Autodesk Inventor part; units mm, degrees
ref_plane "YZ Plane" through (0, 0, 0) normal (1, 0, 0) x (0, 1, 0)
ref_plane "XZ Plane" through (0, 0, 0) normal (0, 1, 0) x (-1, 0, 0)
ref_plane "XY Plane" through (0, 0, 0) normal (0, 0, 1) x (1, 0, 0)
sketch "Sketch1" plane through (0, 0, 0) normal (0, 1, 0) x (-1, 0, 0)
  line L0 (15, 35) -> (-15, 35)
  line L1 (-15, 35) -> (-15, -35)
  line L2 (-15, -35) -> (15, -35)
  line L3 (15, -35) -> (15, 35)
  line L4 (15, 35) -> (-15, -35) construction
  line L5 (-15, 35) -> (15, -35) construction
  point P0 (0, 0)
  dimension "d0" = 30
  dimension "d1" = 70
extrude "gabaryty" add sketch "Sketch1" along normal blind 10
sketch "Sketch2" plane through (0, 10, 0) normal (0, 1, 0) x (1, 0, 0)
  line L0 (5.2, -26) -> (-5.2, -26)
  line L1 (-5.2, -26) -> (-5.2, 26)
  line L2 (-5.2, 26) -> (5.2, 26)
  line L3 (5.2, 26) -> (5.2, -26)
  line L4 (5.2, -26) -> (-5.2, 26) construction
  line L5 (-5.2, -26) -> (5.2, 26) construction
  point P0 (0, 0)
  dimension "d4" = 10.4
  dimension "d5" = 52
extrude "przestrzen srodek" cut sketch "Sketch2" against normal through all
sketch "Sketch3" plane through (0, 10, 0) normal (0, 1, 0) x (1, 0, 0)
  line L0 (5, 5) -> (-5, 5)
  line L1 (-5, 5) -> (-5, -5)
  line L2 (-5, -5) -> (5, -5)
  line L3 (5, -5) -> (5, 5)
  line L4 (5, 5) -> (-5, -5) construction
  line L5 (-5, 5) -> (5, -5) construction
  point P0 (0, 0)
  dimension "d8" = 10
  dimension "d9" = 10
extrude "bloczek srodek" add sketch "Sketch3" against normal blind 10
sketch "Sketch4" plane through (0, 10, 0) normal (0, 1, 0) x (1, 0, 0)
  line L0 (-5, 5) -> (-5, -5) construction
  line L1 (-5, -5) -> (5, -5) construction
  line L2 (5, -5) -> (5, 5) construction
  line L3 (5, 5) -> (-5, 5) construction
  line L4 (-5.2, -26) -> (-5.2, 26) construction
  line L5 (-5.2, 26) -> (5.2, 26) construction
  line L6 (5.2, 26) -> (5.2, -26) construction
  line L7 (5.2, -26) -> (-5.2, -26) construction
  line L8 (15, -35) -> (15, 35) construction
  line L9 (15, 35) -> (-15, 35) construction
  line L10 (-15, 35) -> (-15, -35) construction
  line L11 (-15, -35) -> (15, -35) construction
  line L12 (-5.2, -26) -> (5.2, -26)
  line L13 (-3, -5) -> (-2.6, -5)
  line L14 (-2.6, -5) -> (-2.6, -26)
  line L15 (-2.6, -26) -> (-3, -26)
  line L16 (-3, -26) -> (-3, -5)
  line L17 (3, -5) -> (2.6, -5)
  line L18 (2.6, -5) -> (2.6, -26)
  line L19 (2.6, -26) -> (3, -26)
  line L20 (3, -26) -> (3, -5)
  line L21 (3, 5) -> (2.6, 5)
  line L22 (2.6, 5) -> (2.6, 26)
  line L23 (2.6, 26) -> (3, 26)
  line L24 (3, 26) -> (3, 5)
  line L25 (-5, 5) -> (5, 5)
  line L26 (-3, 5) -> (-2.6, 5)
  line L27 (-2.6, 5) -> (-2.6, 26)
  line L28 (-2.6, 26) -> (-3, 26)
  line L29 (-3, 26) -> (-3, 5)
  point P0 (0, 0)
  point P1 (-2.6, 5)
  dimension "d12" = 0.4
  dimension "d13" = 2
  dimension "d14" = 0.4
  dimension "d15" = 2
  dimension "d16" = 0.4
  dimension "d17" = 2
  dimension "d18" = 0.4
  dimension "d19" = 2
extrude "Belki" add sketch "Sketch4" against normal blind 10
sketch "Sketch5" plane through (0, 10, 0) normal (0, 1, 0) x (1, 0, 0)
  point P0 (0, 0)
  point P1 (0, 0)
hole "srodek" at (0, 10, 0) direction (0, -1, 0) diameter 5.5 end through all
sketch "Sketch6" plane through (-15, 0, -35) normal (-1, 0, 0) x (0, 0, 1)
  line L0 (0, 0) -> (70, 0) construction
  line L1 (70, 0) -> (70, 10) construction
  line L2 (0, 10) -> (70, 10) construction
  line L3 (0, 0) -> (0, 10) construction
  line L4 (35, 0) -> (35, 10) construction
  point P0 (45, 5)
  point P1 (25, 5)
  dimension "d29" = 10
  dimension "d30" = 10
  dimension "d31" = 5
  dimension "d32" = 5
hole "mocowanie gora" at (-15, 5, 10) at (-15, 5, -10) direction (1, 0, 0) diameter 2.459 depth 9.8
chamfer "Chamfer1" distance 0.5 angle 45 2 edges at (-15, 5, -11.2295) (-15, 5, 8.7705)
fillet "zaokraglenie lasera" radius 0.1 24 edges at (-3, 5, 5) (-2.6, 5, 5) (-3, 5, 26) (-2.6, 5, 26) (2.6, 5, 26) (2.6, 5, 5) (3, 5, 5) (3, 5, 26) (3, 5, -5) (2.6, 5, -5) (-2.6, 5, -5) (-3, 5, -5) (-3, 5, -26) (2.6, 5, -26) (-2.6, 5, -26) (3, 5, -26) (-5.2, 5, 26) (-5.2, 5, -26) (5.2, 5, -26) (5.2, 5, 26) (-5, 5, 5) (-5, 5, -5) (5, 5, -5) (5, 5, 5)
chamfer "Chamfer2" distance 0.2 angle 45 1 edges at (0, 10, -2.75)
equation "\"d14\" = d12"
equation "\"d15\" = d13"
equation "\"d16\" = d12"
equation "\"d17\" = d13"
equation "\"d18\" = d12"
equation "\"d19\" = d13"
properties material "Steel ASTM A36"
Part model, mm, in its own coordinate system. A direction names the side the tool comes from. Coordinates: 2 decimals unless noted, no trailing zeros. Write each loop counter-clockwise with the first axis right and the second up, starting at its lowest first coordinate (ties: lowest second). Pieces come first, ordered by that corner, then holes. Notation, with made-up numbers: M 34.25,9 L 60.25,9 A17 ccw 60.25,24 Z; hole C -10,-39 d3. An arc over 180 degrees is marked long. Return JSON: item names as keys, results as strings.
1. Probe L1, parallel to Z at x = 4.5, y = 4; L2, parallel to X at y = 3.25, z = -6.5; L3, parallel to Z at x = -10, y = 5. List the from-to ranges inside material, lowest first.
Determined:
{"L1": "-35 to -26, -5 to 5, 26 to 35", "L2": "-15 to -5.2, -3 to -2.6, 2.6 to 3, 5.2 to 15", "L3": "-35 to -11.23, -8.77 to 8.77, 11.23 to 35"}
2. Pull direction Z, two halves, no side cores. Call faces 1 (the face through (2.6, 5, -15)), 2 (the face through (-4, 10, 0)): pulls with the +Z half, pulls with the -Z half, needs draft (parallel to the pull), parting line crosses it, or undercut.
Determined:
{"face 1": "undercut", "face 2": "needs draft"}
3. Saw through at B-B, the plane z = -6.5. Write the cut outline in (x, y), then the cut area to 3 significant figures.
Determined:
{"outline": "M -15,0 L -5.2,0 L -5.2,10 L -15,10 Z; M -3,0 L -2.6,0 L -2.6,10 L -3,10 Z; M 2.6,0 L 3,0 L 3,10 L 2.6,10 Z; M 5.2,0 L 15,0 L 15,10 L 5.2,10 Z", "area": "204 mm²"}
4. Saw through at C-C, the plane x = 0. Write the cut outline in (y, z).
Determined:
{"outline": "M 0,-35 L 10,-35 L 10,-26 L 0,-26 Z; M 0,-5 L 10,-5 L 10,-2.95 L 9.8,-2.75 L 0,-2.75 Z; M 0,2.75 L 9.8,2.75 L 10,2.95 L 10,5 L 0,5 Z; M 0,26 L 10,26 L 10,35 L 0,35 Z"}
5. 3-axis set-ups, long thin cutter, end or side, ignore diameter. For faces 3 (the face through (0, 5, -26)), 4 (the face through (-9.785, 5.471, 11.136)): which of +Z, -Z, +X, -X, +Y, -Y reach the whole face in a straight line?
Determined:
{"face 3": "+Y, -Y", "face 4": "-X"}
6. Saw through at D-D, the plane y = 5. Count the separate pieces of the cut face and the enclosed holes in it, then the cut area to 3 significant figures.
Determined:
{"separate pieces": "2", "enclosed holes": "4", "area": "1,620 mm²"}
7. Flat gauge pins, fed straight in: pin 1 Ø2 at (x, z) = (-1.5, -14.5) entering from -Y; pin 2 Ø10 at (x, z) = (0, 15) entering from -Y. Where does each tip first touch, or does it go through?
Determined:
{"pin 1": "through", "pin 2": "y = 0"}
8. Saw through at A-A, the plane z = 10. Write the cut outline in (x, y), then the cut area to 3 significant figures.
Determined:
{"outline": "M -15,0 L -5.2,0 L -5.2,3.77 L -14.5,3.77 L -15,3.27 Z; M -15,6.73 L -14.5,6.23 L -5.2,6.23 L -5.2,10 L -15,10 Z; M -3,0 L -2.6,0 L -2.6,10 L -3,10 Z; M 2.6,0 L 3,0 L 3,10 L 2.6,10 Z; M 5.2,0 L 15,0 L 15,10 L 5.2,10 Z", "area": "180 mm²"}
